Could you check a few things on this model? Use its own coordinates, in mm. Face numbers are marked on the shaded views. A direction names the side the tool comes from. Give positions to 0.01 mm unless a question says otherwise; leave off trailing zeros. Write each loop counter-clockwise with the first axis right and the second up, starting at its lowest first coordinate (ties: lowest second). Pieces come first, ordered by that corner, then holes. Notation, with made-up numbers: (69.5, 14) - (95.5, 14) arc R28 ccw to (95.5, 39) - close; hole circle Ø3 at (76, 89.25). An arc over 180 degrees is marked (long way). Write item = value, one per line.
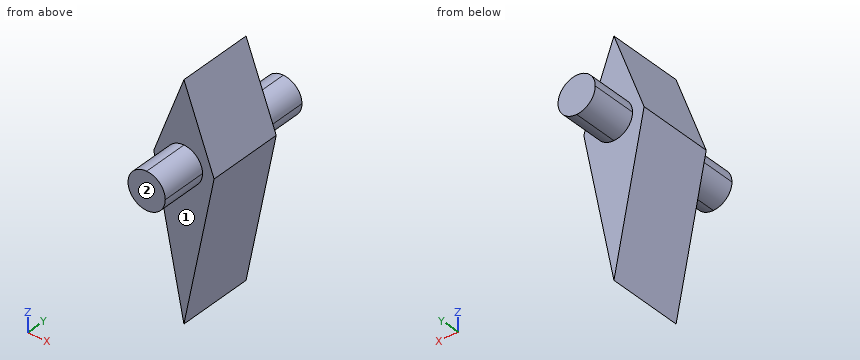
from build123d import *

# Parameters (mm, degrees)
F1_DEPTH      = 7.5
F2_DEPTH      = 12
F2_DEPTH_BACK = 4.5


with BuildPart() as f1:
    # F0 (on Front) → F1 (new body)
    with BuildSketch(Plane.XZ):
        with BuildLine():
            Line((2.9999999901, -0.0002442856), (1.8499999939, -0.0001506428))
            ThreePointArc((1.8499999939, -0.0001506428), (1.3080410203, -1.3082540614), (-0.0001506428, -1.8499999939))
            Line((-0.0001506428, -1.8499999939), (-0.0012214281, -14.9999999503))
            Line((-0.0012214281, -14.9999999503), (2.9999999901, -0.0002442856))
        make_face()
        with BuildLine():
            ThreePointArc((-0.0001506428, -1.8499999939), (-1.3082540614, -1.3080410203), (-1.8499999939, 0.0001506428))
            Line((-1.8499999939, 0.0001506428), (-2.9999999901, 0.0002442856))
            Line((-2.9999999901, 0.0002442856), (-0.0012214281, -14.9999999503))
            Line((-0.0012214281, -14.9999999503), (-0.0001506428, -1.8499999939))
        make_face()
        with BuildLine():
            Line((0, 0), (-1.8499999939, 0.0001506428))
            ThreePointArc((-1.8499999939, 0.0001506428), (-1.3082540614, -1.3080410203), (-0.0001506428, -1.8499999939))
            Line((-0.0001506428, -1.8499999939), (0, 0))
        make_face()
        with BuildLine():
            ThreePointArc((-0.0001506428, -1.8499999939), (1.3080410203, -1.3082540614), (1.8499999939, -0.0001506428))
            Line((1.8499999939, -0.0001506428), (0, 0))
            Line((0, 0), (-0.0001506428, -1.8499999939))
        make_face()
        with BuildLine():
            ThreePointArc((1.8499999939, -0.0001506428), (1.8499999985, -7.53214e-05), (1.85, 0))
            ThreePointArc((1.85, 0), (1.3081475452, 1.3081475452), (0, 1.85))
            Line((0, 1.85), (0, 0))
            Line((0, 0), (1.8499999939, -0.0001506428))
        make_face()
        with BuildLine():
            Line((0, 0), (0, 1.85))
            ThreePointArc((0, 1.85), (-1.3080942838, 1.3082008044), (-1.8499999939, 0.0001506428))
            Line((-1.8499999939, 0.0001506428), (0, 0))
        make_face()
        with BuildLine():
            ThreePointArc((-1.8499999939, 0.0001506428), (-1.3080942838, 1.3082008044), (0, 1.85))
            Line((0, 1.85), (0, 8))
            Line((0, 8), (-2.9999999901, 0.0002442856))
            Line((-2.9999999901, 0.0002442856), (-1.8499999939, 0.0001506428))
        make_face()
        with BuildLine():
            ThreePointArc((0, 1.85), (1.3081475452, 1.3081475452), (1.85, 0))
            ThreePointArc((1.85, 0), (1.8499999985, -7.53214e-05), (1.8499999939, -0.0001506428))
            Line((1.8499999939, -0.0001506428), (2.9999999901, -0.0002442856))
            Line((2.9999999901, -0.0002442856), (0, 8))
            Line((0, 8), (0, 1.85))
        make_face()
    extrude(amount=F1_DEPTH)

    # F0 (on Front) → F2 (join, two sides)
    with BuildSketch(Plane.XZ) as f2_sk:
        with BuildLine():
            Line((0, 0), (-1.8499999939, 0.0001506428))
            ThreePointArc((-1.8499999939, 0.0001506428), (-1.3082540614, -1.3080410203), (-0.0001506428, -1.8499999939))
            Line((-0.0001506428, -1.8499999939), (0, 0))
        make_face()
        with BuildLine():
            Line((0, 0), (0, 1.85))
            ThreePointArc((0, 1.85), (-1.3080942838, 1.3082008044), (-1.8499999939, 0.0001506428))
            Line((-1.8499999939, 0.0001506428), (0, 0))
        make_face()
        with BuildLine():
            ThreePointArc((1.8499999939, -0.0001506428), (1.8499999985, -7.53214e-05), (1.85, 0))
            ThreePointArc((1.85, 0), (1.3081475452, 1.3081475452), (0, 1.85))
            Line((0, 1.85), (0, 0))
            Line((0, 0), (1.8499999939, -0.0001506428))
        make_face()
        with BuildLine():
            ThreePointArc((-0.0001506428, -1.8499999939), (1.3080410203, -1.3082540614), (1.8499999939, -0.0001506428))
            Line((1.8499999939, -0.0001506428), (0, 0))
            Line((0, 0), (-0.0001506428, -1.8499999939))
        make_face()
    extrude(amount=F2_DEPTH)
    extrude(f2_sk.sketch, amount=-F2_DEPTH_BACK)


solid = f1.part
1. For pin 1 (4 mm diameter, centred on y = -5.5, z = 4.5, fed in from -X); pin 2 (1.5 mm diameter, centred on x = 0.5, y = 2, fed in from -Z); pin 3 (8 mm diameter, centred on y = -5, z = 5.5, fed in from +X), each with a flat end and sliding along its axis, tell me the tip position at first contact or that it passes through.
Filled sheet:
pin_1 = -2.06
pin_2 = -1.85
pin_3 = 2.44
2. Which directions (+Z, -Z, +X, -X, +Y, -Y) give clear straight access to the entire face, cutting with the end or side of a thin tool? Please do the marked faces 1 and 2.
Filled sheet:
face_1 = -Y
face_2 = +Z, -Z, +X, -X, -Y
3. If we section it at B-B, the plane z = 0.75: Please give me the cut outline in (x, y).
Filled sheet:
outline = (-2.72, -7.5) - (-1.69, -7.5) - (-1.69, -12) - (1.69, -12) - (1.69, -7.5) - (2.72, -7.5) - (2.72, 0) - (1.69, 0) - (1.69, 4.5) - (-1.69, 4.5) - (-1.69, 0) - (-2.72, 0) - close
4. I need wall thicknesses on line 1 (X direction, y = -6.75, z = -5.75); line 2 (Y direction, x = 0.1, z = -11.25). Which ranges of each line are inside material? Lowest first, please.
Filled sheet:
line_1 = -1.85 to 1.85
line_2 = -7.5 to 0
5. If we section it at D-D, the plane z = -9.25: Please give me the cut outline in (x, y), and give its area (4 significant figures).
Filled sheet:
outline = (-1.15, -7.5) - (1.15, -7.5) - (1.15, 0) - (-1.15, 0) - close
area = 17.25 mm2
6. If we section it at A-A, the plane x = -1.5: Please give me the cut outline in (y, z), and give its area (3 significant figures).
Filled sheet:
outline = (-12, -1.08) - (-7.5, -1.08) - (-7.5, -7.5) - (0, -7.5) - (0, -1.08) - (4.5, -1.08) - (4.5, 1.08) - (0, 1.08) - (0, 4) - (-7.5, 4) - (-7.5, 1.08) - (-12, 1.08) - close
area = 106 mm2
